Part model, mm, in its own coordinate system. Give positions to 0.01 mm unless a question says otherwise; leave off trailing zeros. Order: outer loops, then holes, each group sorted by start corner. A loop starts at its lowest first (then second) coordinate and runs counter-clockwise, first axis right, second up. Notation, with made-up numbers: (-29, -12) - (-8, -12) arc R7 ccw to (-8, -5) - close; hole circle Ø6 at (80, 72.5). An arc over 180 degrees is marked (long way). One line per item, written item: value.
```python
from build123d import *

# Parameters (mm, degrees)
SKETCH2_W           = 110
SKETCH2_H           = 16
BOSS_EXTRUDE1_DEPTH = 5
SKETCH3_R           = 3
CUT_EXTRUDE1_DEPTH  = 56.803225713
SKETCH5_R           = 2
CUT_EXTRUDE2_DEPTH  = 56.803225713
FILLET1_R           = 8
FILLET2_R           = 1


with BuildPart() as part:
    # Sketch2 → Boss-Extrude1 (new body)
    with BuildSketch(Plane(origin=(0, 0, 0), x_dir=(1, 0, 0), z_dir=(0, 1, 0))):
        Rectangle(SKETCH2_W, SKETCH2_H)
    extrude(amount=BOSS_EXTRUDE1_DEPTH)

    # Sketch3 → Cut-Extrude1 (cut, through all)
    with BuildSketch(Plane(origin=(0, 5, 0), x_dir=(1, 0, 0), z_dir=(0, 1, 0))):
        with Locations(Location((-43, 0, 0), (0, 0, 270))):
            Circle(SKETCH3_R)
    extrude(amount=-CUT_EXTRUDE1_DEPTH, mode=Mode.SUBTRACT)

    # Sketch5 → Cut-Extrude2 (cut, through all)
    with BuildSketch(Plane(origin=(0, 5, 0), x_dir=(1, 0, 0), z_dir=(0, 1, 0))):
        with Locations(Location((-15, 0, 0), (0, 0, 270))):
            Circle(SKETCH5_R)
        with Locations(Location((5, 0, 0), (0, 0, 270))):
            Circle(SKETCH5_R)
        with Locations(Location((25, 0, 0), (0, 0, 270))):
            Circle(SKETCH5_R)
        with Locations(Location((45, 0, 0), (0, 0, 270))):
            Circle(SKETCH5_R)
    extrude(amount=-CUT_EXTRUDE2_DEPTH, mode=Mode.SUBTRACT)

    # Fillet1
    # the kernel refuses this fillet: 8 mm, written as the material it takes off along each edge
    with BuildSketch(Plane(origin=(55, 5, -26.540496218), x_dir=(0, -1, 0), z_dir=(0, 0, 1)), Plane(origin=(-55, 5, 26.540496218), x_dir=(0, -1, 0), z_dir=(0, 0, -1))) as fillet1_piece_1:
        with BuildLine():
            CenterArc((8, -7.416198487), FILLET1_R, 112.024312837, 67.975687163)
            Line((0, -7.416198487), (-0.16, -7.416198487))
            Line((-0.16, -7.416198487), (-0.16, 0))
            Line((-0.16, 0), (0, 0.16))
            ThreePointArc((0, 0.16), (2.5, 0.16), (4.94, 0.14832397))
            Line((4.94, 0.14832397), (5, 0))
        make_face()
    extrude(amount=53.080992435, mode=Mode.SUBTRACT)

    # Fillet2
    fillet2_edges = [part.edges().sort_by_distance(p)[0] for p in [
        (0, 5, -8),
        (0, 5, 8),
        (-52.055937468, 3.633249581, -8),
        (52.055937468, 3.633249581, -8),
        (-52.055937468, 3.633249581, 8),
        (52.055937468, 3.633249581, 8),
        (0, 0, 8),
        (0, 0, -8),
    ]]
    fillet(fillet2_edges, radius=FILLET2_R)


solid = part.part
```
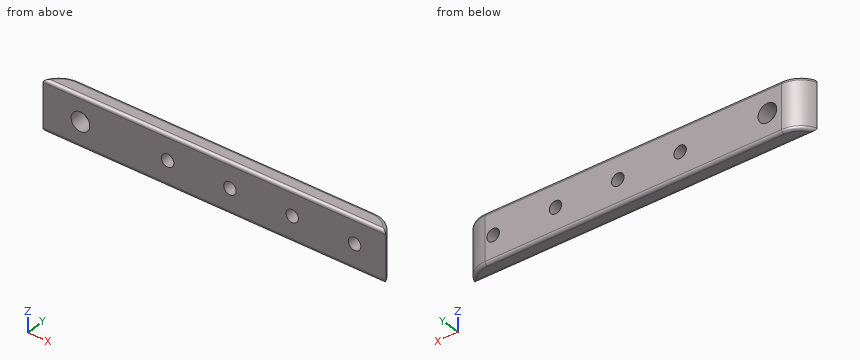
1) Cut at B-B, the plane x = -43. Give the cut face in (y, z).
Outcome:
outline: (0, -7) arc R1 ccw to (1, -8) - (4, -8) arc R1 ccw to (5, -7) - (5, -3) - (0, -3) - close; (0, 3) - (5, 3) - (5, 7) arc R1 ccw to (4, 8) - (1, 8) arc R1 ccw to (0, 7) - close
2) Drill centre lines: line 1 along X through (y, z) = (2.6, 0); line 2 along X through (y, z) = (1.6, 0); line 3 along X through (y, z) = (2.3, 7.25). Where is each one in solid material? Low to high. Write a range as from..to.
Outcome:
line 1: x = -53.3..-46, -40..-17, -13..3, 7..23, 27..43, 47..53.3
line 2: x = -54.13..-46, -40..-17, -13..3, 7..23, 27..43, 47..54.13
line 3: x = -53.53..53.53
3) Cut at D-D, the plane y = 2.25. Give the number of separate pieces and of enclosed holes in the cut face, then the cut area to 3 significant figures.
Outcome:
separate pieces: 1
enclosed holes: 5
area: 1,640 mm^2
4) Cut at A-A, the plane x = 5. Give the cut face in (y, z).
Outcome:
outline: (0, -7) arc R1 ccw to (1, -8) - (4, -8) arc R1 ccw to (5, -7) - (5, -2) - (0, -2) - close; (0, 2) - (5, 2) - (5, 7) arc R1 ccw to (4, 8) - (1, 8) arc R1 ccw to (0, 7) - close
5) Pin check, flat tips, straight feed: pin 1 (1 mm diameter, centred on y = 1, z = 5, fed in from -X); pin 2 (3 mm diameter, centred on x = 5, z = 0, fed in from +Y). Stop position of each tip, or through.
Outcome:
pin 1: stops at x = -54.78
pin 2: passes through
6) Cut at C-C, the plane z = -4.75. Give the cut face in (x, y).
Outcome:
outline: (-55, 0) - (55, 0) arc R8 ccw to (47.58, 5) - (-47.58, 5) arc R8 ccw to start
